Geometry: final body of the model. Coordinates: model frame, mm. A direction names the side the tool comes from. Round coordinates to 2 decimals unless told otherwise and drop trailing zeros. Loops run counter-clockwise (first coordinate to the right, second up) from the corner with the lowest first, then second, coordinate; pieces in that order, holes last. Notation, with made-up numbers: (50.5, 54) - (81.5, 54) arc R20 cw to (81.5, 74) - close; hole circle Ø5 at (-16, 78). An arc over 180 degrees is marked (long way). Use CSV: the item, a comma, the result in double quotes.
from build123d import *

# Parameters (mm, degrees)
SKETCH256_R             = 1.45
PAD243_DEPTH            = 10.4
SKETCH257_W             = 2.9
SKETCH257_H             = 4.1
PAD244_DEPTH            = 3
SKETCH258_W             = 0.8
SKETCH258_H             = 6.4
PAD245_DEPTH            = 10
PAD246_DEPTH            = 3
BODY085_PLACEMENT_ANGLE = 90
PAD242_DEPTH            = 11


with BuildPart() as body086:
    # Sketch260 → Revolution010 (revolve)
    with BuildSketch(Plane.XY):
        Polygon((5.19, 1.5), (-5.19, 1.5), (-4.79, 0.928741), (-4.79, 0), (4.79, 0), (4.79, 0.928741), align=None)
    revolve(axis=Axis((0, 0, 0), (1, 0, 0)))


with BuildPart() as body086_1:
    # Body086 placement: moved
    add(body086.part.moved(Location((9.65, -4.84, 10.9))))


with BuildPart() as switch039:
    # Sketch256 → Pad243 (new body)
    with BuildSketch(Plane.XY):
        with BuildLine():
            ThreePointArc((-12.35, 8.1), (-13.587437, 7.587437), (-14.1, 6.35))
            Line((-14.1, -6.35), (-14.1, 6.35))
            ThreePointArc((-14.1, -6.35), (-13.587437, -7.587437), (-12.35, -8.1))
            Line((12.35, -8.1), (-12.35, -8.1))
            ThreePointArc((12.35, -8.1), (13.587437, -7.587437), (14.1, -6.35))
            Line((14.1, 6.35), (14.1, -6.35))
            ThreePointArc((14.1, 6.35), (13.587437, 7.587437), (12.35, 8.1))
            Line((-12.35, 8.1), (12.35, 8.1))
        make_face()
        with Locations((10.877931, -4.825)):
            Circle(SKETCH256_R, mode=Mode.SUBTRACT)
        with Locations((-10.877931, 4.825)):
            Circle(SKETCH256_R, mode=Mode.SUBTRACT)
    extrude(amount=PAD243_DEPTH)

    # Sketch257 (on Face8 of Pad243) → Pad244 (join)
    with BuildSketch(Plane(origin=(0, 8.1, 0), x_dir=(-1, 0, 0), z_dir=(0, 1, 0))):
        with Locations((-9.45, 5.2)):
            Rectangle(SKETCH257_W, SKETCH257_H)
    extrude(amount=PAD244_DEPTH)

    # Sketch258 (on Face3 of Pad244) → Pad245 (join)
    with BuildSketch(Plane(origin=(-14.1, 0, 0), x_dir=(0, -1, 0), z_dir=(-1, 0, 0))):
        with Locations((4.3, 5.2)):
            Rectangle(SKETCH258_W, SKETCH258_H)
    extrude(amount=PAD245_DEPTH)

    # Sketch259 (on Face16 of Pad245) → Pad246 (join)
    with BuildSketch(Plane.XZ.offset(8.1)):
        Polygon((-3.5, 8.45), (-0.5, 8.45), (-0.5, 1.95), (-3.5, 1.95), (-3.5, 2.7), (-9.5, 2.7), (-9.5, 7.7), (-3.5, 7.7), align=None)
    extrude(amount=PAD246_DEPTH)


with BuildPart() as switch039_1:
    # Body085 placement: moved
    add(switch039.part.moved(Location((14.15, 0, 0))).rotate(Axis((14.15, 0, 0), (0, -1, 0)), BODY085_PLACEMENT_ANGLE))


with BuildPart() as cut028:
    # Sketch255 → Pad242 (new body)
    with BuildSketch(Plane.XZ):
        Polygon((-4, 7.5), (4, 7.5), (6.5, 2.5), (6.5, -12.5), (-6.5, -12.5), (-6.5, 2.5), align=None)
    extrude(amount=PAD242_DEPTH)


with BuildPart() as cut028_1:
    # Body084 placement: moved
    add(cut028.part.moved(Location((8.95, 0, 6.5))))

    # Cut027: cut switch039
    add(switch039_1.part, mode=Mode.SUBTRACT)


with BuildPart() as cut028_2:
    # Cut027 placement: moved
    add(cut028_1.part.moved(Location((0.7, 0, 0))))

    # Cut028: cut Body086
    add(body086_1.part, mode=Mode.SUBTRACT)


solid = cut028_2.part
Item 1: Mould query, pull axis X, two halves, no side actions, for faces 4 (the flat face through (16.15, -5, 2)), 5 (the flat face through (4, -7, -6)), 6 (the flat face through (14.44, -5, 11)), 7 (the flat face through (10, -8.1, 5)). Classes: released by +X, released by -X, zero draft, split by the parting line, or undercut.
Final values:
face 4,"released by +X"
face 5,"zero draft"
face 6,"undercut"
face 7,"undercut"
Item 2: Section A-A on x = 6.75. Return the cut outline in (y, z).
Final values:
outline,"(-11, -6) - (-8.1, -6) - (-8.1, -3.5) - (-11, -3.5) - close; (-11, -0.5) - (-8.1, -0.5) - (-8.1, 12.35) arc R1.75 cw to (-6.93, 14) - (-11, 14) - close"
Item 3: Material intervals for line 1 (X direction, y = -8.75, z = -2.5); line 2 (X direction, y = -7.5, z = 1.5); line 3 (Z direction, x = 12.25, y = -10), sorted ascending.
Final values:
line 1,"x = 3.15 to 6.4, 12.9 to 16.15"
line 2,"x = 3.15 to 4.45, 14.85 to 16.15"
line 3,"z = -6 to -3.5, -0.5 to 14"
Item 4: Reachability of faces 1 (the flat face through (4.86, -5, 11)), 2 (the flat face through (6.4, -10, -2)), 3 (the flat face through (7.15, -10, -5)) from +Z, -Z, +X, -X, +Y, -Y: full face, straight path, thin tool, end or side. Return the list, or none.
Final values:
face 1,"+Z, -Z, +Y"
face 2,"+Y, -Y"
face 3,"-Z, +Y, -Y"
Item 5: Pin query (flat end, axial travel): P1, Ø2, axis at y = -5, z = 11, coming from the -X side; P2, Ø5, axis at x = 9, z = 6, coming from the +Y side; P3, Ø0.9, axis at y = -5, z = 11.5, coming from the +X side (3 decimals). Return the tip coordinate at first contact, or that it passes through.
Final values:
P1,"stops at x = 3.65"
P2,"stops at y = -8.1"
P3,"stops at x = 15.125"
Item 6: Section C-C on z = 4. Return the cut outline in (x, y).
Final values:
outline,"(3.15, -11) - (16.15, -11) - (16.15, 0) - (14.85, 0) - (14.85, -8.1) - (4.45, -8.1) - (4.45, 0) - (3.15, 0) - close"
Item 7: Section B-B on y = -1.75. Return the cut outline in (x, z), plus the area to 3 significant figures.
Final values:
outline,"(3.15, -6) - (4.45, -6) - (4.45, 11.6) - (3.15, 9) - close; (14.85, -6) - (16.15, -6) - (16.15, 9) - (14.85, 11.6) - close"
area,"42.4 mm²"
